Here's how the part is built. I have some questions about the finished solid (model axes, mm). Give positions to 0.01 mm unless a question says otherwise; leave off trailing zeros. Order: outer loops, then holes, each group sorted by start corner. A loop starts at its lowest first (then second) coordinate and runs counter-clockwise, first axis right, second up. Notation, with made-up numbers: (5, -30) -> (53, -30) arc R23 ccw to (53, 9) -> close; hole circle Ø9 at (-10.5, 43.25). An arc over 180 degrees is marked (long way). Write each question's results on one line, items separated by ' | '. Start each with the question number.
Q1. I need wall thicknesses on line 1 along Z through (x, y) = (83.5, 2.2); line 2 along Z through (x, y) = (-5, 1.65); line 3 along Z through (x, y) = (6, 0.9). Which ranges of each line are inside material? Lowest first, please. Write a range as [from, to].
Q2. I'm going to push a flat-ended pin straight in: pin 1 (4 mm diameter, centred on x = -85.035, z = -85.035, fed in from +Y). Where does the tip first touch, or does it pass through?
Q3. Imagine slicing it at A-A, the plane x = 0. Please give me the cut outline in (y, z).
Q4. Imagine slicing it at B-B, the plane z = 32.24. Please give me the cut outline in (x, y), then the cut area to 3 significant figures.
Q5. Thinking about a two-plate mould opening in X: for faces 1 (the face through (0.747, 1.521, 15.256)), 2 (the face through (-2, 3, -2)), which applies, pulls with the +X half, pulls with the -X half, needs draft (parallel to the pull), parting line crosses it, or undercut?
```python
from build123d import *

# Parameters (mm, degrees)
SKETCH2_W           = 304.8
SKETCH2_H           = 304.8
BOSS_EXTRUDE1_DEPTH = 3
SKETCH3_R           = 2.5
CUT_EXTRUDE1_DEPTH  = 216.547025032
SKETCH4_R           = 17
CUT_EXTRUDE2_DEPTH  = 216.547025032


with BuildPart() as part:
    # Sketch2 → Boss-Extrude1 (new body)
    with BuildSketch(Plane(origin=(0, 0, 0), x_dir=(1, 0, 0), z_dir=(0, 1, 0))):
        Rectangle(SKETCH2_W, SKETCH2_H)
    extrude(amount=BOSS_EXTRUDE1_DEPTH)

    # Sketch3 → Cut-Extrude1 (cut, through all)
    with BuildSketch(Plane(origin=(0, 3, 0), x_dir=(1, 0, 0), z_dir=(0, 1, 0))):
        with Locations(Location((-85.035, 85.035, 0), (0, 0, 270))):
            Circle(SKETCH3_R)
        with Locations(Location((85.035, 85.035, 0), (0, 0, 270))):
            Circle(SKETCH3_R)
        with Locations(Location((-85.035, -85.035, 0), (0, 0, 270))):
            Circle(SKETCH3_R)
        with Locations(Location((85.035, -85.035, 0), (0, 0, 270))):
            Circle(SKETCH3_R)
    extrude(amount=-CUT_EXTRUDE1_DEPTH, mode=Mode.SUBTRACT)

    # Sketch4 → Cut-Extrude2 (cut, through all)
    with BuildSketch(Plane(origin=(0, 3, 0), x_dir=(1, 0, 0), z_dir=(0, 1, 0))):
        with Locations(Location((0, -32.24, 0), (0, 0, 270))):
            Circle(SKETCH4_R)
    extrude(amount=-CUT_EXTRUDE2_DEPTH, mode=Mode.SUBTRACT)


solid = part.part
```
Geometry check:
1) line 1: [-152.4, -87.01], [-83.06, 83.06], [87.01, 152.4] | line 2: [-152.4, 15.99], [48.49, 152.4] | line 3: [-152.4, 16.33], [48.15, 152.4]
2) pin 1: through
3) outline: (0, -152.4) -> (3, -152.4) -> (3, 15.24) -> (0, 15.24) -> close; (0, 49.24) -> (3, 49.24) -> (3, 152.4) -> (0, 152.4) -> close
4) outline: (-152.4, 0) -> (-17, 0) -> (-17, 3) -> (-152.4, 3) -> close; (17, 0) -> (152.4, 0) -> (152.4, 3) -> (17, 3) -> close | area: 812 mm²
5) face 1: undercut | face 2: needs draft
